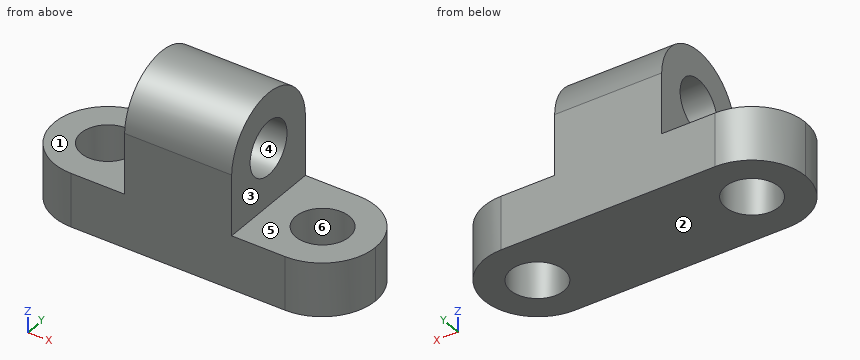
```python
from build123d import *

# Parameters (mm, degrees)
F1_DEPTH  = 25.4
F2_R      = 6.35
F3_DEPTH  = 12.7
F5_DEPTH  = 12.7
F6_R      = 6.35
F7_DEPTH  = 12.7
F9_DEPTH  = 12.7
F10_R     = 6.35
F11_DEPTH = 25.4
F13_DEPTH = 25.4


with BuildPart() as f1:
    # F0 (on Front) → F1 (new body)
    with BuildSketch(Plane.XZ):
        Polygon((0, 12.7), (0, 0), (76.2, 0), (76.2, 12.7), (50.8, 12.7), (50.8, 39.9142862895), (25.4, 39.9142862895), (25.4, 12.7), align=None)
    extrude(amount=F1_DEPTH)

    # F2 (on face) → F3 (cut)
    with BuildSketch(Plane.XY.offset(12.7)):
        with Locations((63.6192816147, -12.6994398261)):
            Circle(F2_R)
    extrude(amount=-F3_DEPTH, mode=Mode.SUBTRACT)

    # F4 (on face) → F5 (cut)
    with BuildSketch(Plane.XY.offset(12.7)):
        with BuildLine():
            ThreePointArc((63.5, 0), (72.4802561211, -3.7197438789), (76.2, -12.7))
            Line((76.2, -12.7), (76.2, 0))
            Line((76.2, 0), (63.5, 0))
        make_face()
        with BuildLine():
            ThreePointArc((76.2, -12.7), (72.4802561211, -21.6802561211), (63.5, -25.4))
            Line((63.5, -25.4), (76.2, -25.4))
            Line((76.2, -25.4), (76.2, -12.7))
        make_face()
    extrude(amount=-F5_DEPTH, mode=Mode.SUBTRACT)

    # F6 (on face) → F7 (cut)
    with BuildSketch(Plane.XY.offset(12.7)):
        with Locations((12.7, -12.7)):
            Circle(F6_R)
    extrude(amount=-F7_DEPTH, mode=Mode.SUBTRACT)

    # F8 (on face) → F9 (cut)
    with BuildSketch(Plane.XY.offset(12.7)):
        with BuildLine():
            ThreePointArc((12.7, -25.4), (3.7197438789, -21.6802561211), (0, -12.7))
            Line((0, -12.7), (0, -25.4))
            Line((0, -25.4), (12.7, -25.4))
        make_face()
        with BuildLine():
            ThreePointArc((0, -12.7), (3.7197438789, -3.7197438789), (12.7, 0))
            Line((12.7, 0), (0, 0))
            Line((0, 0), (0, -12.7))
        make_face()
    extrude(amount=-F9_DEPTH, mode=Mode.SUBTRACT)

    # F10 (on face) → F11 (cut)
    with BuildSketch(Plane.YZ.offset(50.8)):
        with Locations((-12.7, 26.3071431448)):
            Circle(F10_R)
    extrude(amount=-F11_DEPTH, mode=Mode.SUBTRACT)

    # F12 (on face) → F13 (cut)
    with BuildSketch(Plane.YZ.offset(50.8)):
        with BuildLine():
            ThreePointArc((-25.4, 27.0906584082), (-12.7, 39.4049416249), (0, 27.0906584082))
            Line((0, 27.0906584082), (0, 39.9142862895))
            Line((0, 39.9142862895), (-25.4, 39.9142862895))
            Line((-25.4, 39.9142862895), (-25.4, 27.0906584082))
        make_face()
    extrude(amount=-F13_DEPTH, mode=Mode.SUBTRACT)


solid = f1.part
```
Could you check a few things on this model? Use its own coordinates, in mm. Face numbers are marked on the shaded views. A direction names the side the tool comes from. Round coordinates to 2 decimals unless told otherwise and drop trailing zeros. Loops run counter-clockwise (first coordinate to the right, second up) from the corner with the lowest first, then second, coordinate; pieces in that order, holes last. Notation, with made-up numbers: (75, 87) - (113, 87) arc R4 ccw to (113, 91) - close; hole circle Ø2 at (18, -23). An arc over 180 degrees is marked (long way). Use CSV: the item, a comma, the result in double quotes.
Item 1: For the marked faces 1, 2 and 3, which set-ups out of +Z, -Z, +X, -X, +Y, -Y let a thin tool reach every point of the face, with its end or its side?
Here are the results:
face 1,"+Z, -X, +Y, -Y"
face 2,"-Z, +X, -X, +Y, -Y"
face 3,"+Z, +X, +Y, -Y"
Item 2: If we section it at A-A on y = -13.5: List the corners of the cut face in (x, z) for me, then the cut area to 3 significant figures.
Here are the results:
outline,"(0.03, 0) - (6.4, 0) - (6.4, 12.7) - (0.03, 12.7) - close; (19, 0) - (57.32, 0) - (57.32, 12.7) - (50.8, 12.7) - (50.8, 20.01) - (25.4, 20.01) - (25.4, 12.7) - (19, 12.7) - close; (25.4, 32.61) - (50.8, 32.61) - (50.8, 39.38) - (25.4, 39.38) - close; (69.92, 0) - (76.17, 0) - (76.17, 12.7) - (69.92, 12.7) - close"
area,"1,000 mm²"
Item 3: If we section it at C-C on x = 41.5: List the corners of the cut face in (y, z) for me.
Here are the results:
outline,"(-25.4, 0) - (0, 0) - (0, 27.09) arc R12.71 ccw to (-25.4, 27.09) - close; hole circle Ø12.7 at (-12.7, 26.31)"
Item 4: If we section it at D-D on y = -23: List the corners of the cut face in (x, z) for me, then the cut area to 3 significant figures.
Here are the results:
outline,"(5.27, 0) - (70.93, 0) - (70.93, 12.7) - (50.8, 12.7) - (50.8, 34.14) - (25.4, 34.14) - (25.4, 12.7) - (5.27, 12.7) - close"
area,"1,380 mm²"
Item 5: I need wall thicknesses on L1, parallel to Y at x = 12.7, z = 3.75; L2, parallel to X at y = -10.5, z = 10; L3, parallel to Z at x = 57, y = -5.75. Which ranges of each line are inside material? Lowest first, please. Write a range as [from, to].
Here are the results:
L1,"y = [-25.4, -19.05], [-6.35, 0]"
L2,"x = [0.19, 6.74], [18.66, 57.66], [69.58, 76.01]"
L3,"z = [0, 12.7]"
Item 6: If we section it at B-B on x = 59: List the corners of the cut face in (y, z) for me, then the cut area to 3 significant figures.
Here are the results:
outline,"(-25.4, 0) - (-17.06, 0) - (-17.06, 12.7) - (-25.4, 12.7) - close; (-8.34, 0) - (0, 0) - (0, 12.7) - (-8.34, 12.7) - close"
area,"212 mm²"
Item 7: Will these pins go through, and if not, where does the flat tip stop? pin 1 (12.5 mm diameter, centred on y = -7, z = 22, fed in from +X); pin 2 (10 mm diameter, centred on x = 12.7, y = -12.7, fed in from +Z); pin 3 (8 mm diameter, centred on y = -14.5, z = 29, fed in from -X); pin 4 (7.5 mm diameter, centred on x = 15.5, y = -12.5, fed in from +Z).
Here are the results:
pin 1,"stops at x = 50.8"
pin 2,"passes through"
pin 3,"stops at x = 25.4"
pin 4,"stops at z = 12.7"
Item 8: If we mould it in two halves opening along Z, with no side actions, what happens to the marked faces 4, 5 and 6? For each: pulls with the +Z half, pulls with the -Z half, needs draft (parallel to the pull), parting line crosses it, or undercut.
Here are the results:
face 4,"undercut"
face 5,"pulls with the +Z half"
face 6,"needs draft"
